from build123d import *

# Parameters (mm, degrees)
BOSS_EXTRUDE1_DEPTH = 100
SKETCH3_R           = 14.75
SKETCH3_R_2         = 2.75
BOSS_EXTRUDE2_DEPTH = 8
SKETCH4_R           = 8.075
CUT_EXTRUDE1_DEPTH  = 5.2
BOSS_EXTRUDE5_START = 11
SKETCH6_R           = 2.25
BOSS_EXTRUDE5_DEPTH = 4.5
BOSS_EXTRUDE6_DEPTH = 3


with BuildPart() as part:
    # Sketch1 → Boss-Extrude1 (new body, symmetric)
    with BuildSketch(Plane.YZ):
        with BuildLine():
            Line((-24.5, 5), (-24.5, -5))
            Line((-24.5, -5), (24.5, -5))
            Line((24.5, -5), (24.5, 5))
            Line((24.5, 5), (16.492422502, 5))
            ThreePointArc((16.492422502, 5), (0, -3), (-16.492422502, 5))
            Line((-16.492422502, 5), (-24.5, 5))
        make_face()
    extrude(amount=BOSS_EXTRUDE1_DEPTH, both=True)

    # Sketch3 → Boss-Extrude2 (add)
    with BuildSketch(Plane.XZ.offset(24.5)):
        with Locations((0, -19.75)):
            Circle(SKETCH3_R)
        with Locations((0, -19.75)):
            Circle(SKETCH3_R_2, mode=Mode.SUBTRACT)
        with BuildLine():
            Line((-14.75, -5), (-14.75, -19.75))
            ThreePointArc((-14.75, -19.75), (-10.429825021, -9.320174976), (5e-09, -5))
            Line((5e-09, -5), (-14.75, -5))
        make_face()
        with BuildLine():
            ThreePointArc((5e-09, -5), (10.429825024, -9.320174979), (14.75, -19.75))
            Line((14.75, -19.75), (14.75, -5))
            Line((14.75, -5), (5e-09, -5))
        make_face()
    boss_extrude2 = extrude(amount=-BOSS_EXTRUDE2_DEPTH)

    # Sketch4 → Cut-Extrude1 (cut)
    with BuildSketch(Plane(origin=(0, -24.5, 0), x_dir=(-1, 0, 0), z_dir=(0, -1, 0))):
        with Locations((0, 19.75)):
            Circle(SKETCH4_R)
    cut_extrude1 = extrude(amount=-CUT_EXTRUDE1_DEPTH, mode=Mode.SUBTRACT)

    # Mirror1: Boss-Extrude2, Cut-Extrude1 across plane
    add(boss_extrude2.mirror(Plane(origin=(0, 0, 0), x_dir=(0, 0, 1), z_dir=(0, -1, 0))))
    add(cut_extrude1.mirror(Plane(origin=(0, 0, 0), x_dir=(0, 0, 1), z_dir=(0, -1, 0))), mode=Mode.SUBTRACT)

    # Sketch6 → Boss-Extrude5 (add)
    with BuildSketch(Plane(origin=(0, 0, 0), x_dir=(-1, 0, 0), z_dir=(0, -1, 0)).offset(BOSS_EXTRUDE5_START)):
        with BuildLine():
            Line((87.25, 19.75), (87.25, 5))
            Line((87.25, 5), (97.75, 5))
            Line((97.75, 5), (97.75, 19.75))
            ThreePointArc((97.75, 19.75), (92.5, 25), (87.25, 19.75))
        make_face()
        with Locations((92.5, 19.75)):
            Circle(SKETCH6_R, mode=Mode.SUBTRACT)
    boss_extrude5 = extrude(amount=BOSS_EXTRUDE5_DEPTH)

    # Mirror2: Boss-Extrude5 across plane
    add(boss_extrude5.mirror(Plane(origin=(0, 0, 0), x_dir=(0, 0, 1), z_dir=(0, -1, 0))))

    # Sketch7 → Boss-Extrude6 (add)
    with BuildSketch(Plane(origin=(-100, 0, 0), x_dir=(0, -1, 0), z_dir=(-1, 0, 0))):
        with BuildLine():
            Line((24.5, 5), (16.492422502, 5))
            ThreePointArc((16.492422502, 5), (0, -3), (-16.492422502, 5))
            Line((-16.492422502, 5), (-24.5, 5))
            Line((-24.5, 5), (-24.5, -5))
            Line((-24.5, -5), (24.5, -5))
            Line((24.5, -5), (24.5, 5))
        make_face()
        with BuildLine():
            Line((-16.492422502, 5), (16.492422502, 5))
            ThreePointArc((16.492422502, 5), (0, -3), (-16.492422502, 5))
        make_face()
        with BuildLine():
            ThreePointArc((24.5, 5), (0, 13), (-24.5, 5))
            Line((-24.5, 5), (-16.492422502, 5))
            Line((-16.492422502, 5), (16.492422502, 5))
            Line((16.492422502, 5), (24.5, 5))
        make_face()
    boss_extrude6 = extrude(amount=-BOSS_EXTRUDE6_DEPTH)

    # Mirror3: Boss-Extrude6 across plane
    add(boss_extrude6.mirror(Plane(origin=(0, 0, 0), x_dir=(0, 0, 1), z_dir=(1, 0, 0))))


solid = part.part
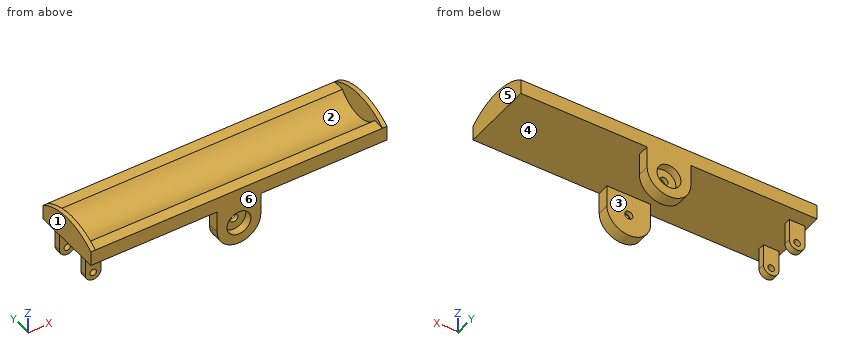
Work out the finished part from the listing and answer in its coordinate system (mm). Face numbers are marked on the shaded views. A direction names the side the tool comes from. Round coordinates to 2 decimals unless told otherwise and drop trailing zeros. Order: outer loops, then holes, each group sorted by start corner. A loop starts at its lowest first (then second) coordinate and runs counter-clockwise, first axis right, second up. Notation, with made-up numbers: M 10.25,-16.5 L 22.25,-16.5 A23 ccw 22.25,0.5 Z; hole C -5,-24 d3. An arc over 180 degrees is marked long. Put each result on its own line as item: value. Start each with the question number.
Q1. Section A-A, the plane x = -92.5 is taken. Write down the section's boundary in (y, z), and give its area (3 significant figures).
Q2. Section C-C, the plane x = -57 is taken. Write down the section's boundary in (y, z), and give its area (3 significant figures).
Q3. A tool of negligible diameter and unlimited length cuts with its end or side. For the marked faces 1, 2 and 3, from which of +Z, -Z, +X, -X, +Y, -Y can it reach the whole face along a straight path? Write none if from no direction.
Q4. Section B-B, the plane z = 7 is taken. Write down the section's boundary in (x, y), and give its area (3 significant figures).
Q5. Flat-ended cylindrical pins translate along their axes: pin 1 (6 mm diameter, centred on x = -92.5, z = -19.75, fed in from -Y); pin 2 (2.5 mm diameter, centred on y = 20, z = -13, fed in from -X); pin 3 (1.3 mm diameter, centred on y = -13.5, z = -15, fed in from -X); pin 4 (11.5 mm diameter, centred on x = -92, z = -10.5, fed in from +Y). Find the tip coordinate at first contact, or state that the pin passes through.
Q6. For a pull along Y with two mould halves and no side action, classify the marked faces 4, 5 and 6 as pulls with the +Y half, pulls with the -Y half, needs draft (parallel to the pull), parting line crosses it, or undercut.
Q7. Section D-D, the plane x = 0 is taken. Write down the section's boundary in (y, z) (3 decimals).
Q8. Straight lines are drawn through the part: L1, parallel to Z at x = 0, y = 18.65; L2, parallel to X at y = -22.8, z = -19.75 (3 decimals); L3, parallel to Y at x = 2.5, z = -13. For each, find the intervals that lie inside material, in ascending order. Write a range as [from, to].
Findings below:
1. outline: M -24.5,-5 L -15.5,-5 L -15.5,-17.5 L -11,-17.5 L -11,-5 L 11,-5 L 11,-17.5 L 15.5,-17.5 L 15.5,-5 L 24.5,-5 L 24.5,5 L 16.49,5 A21 cw -16.49,5 L -24.5,5 Z; M -15.5,-25 L -11,-25 L -11,-22 L -15.5,-22 Z; M 11,-25 L 15.5,-25 L 15.5,-22 L 11,-22 Z
1. area: 446 mm^2
2. outline: M -24.5,-5 L 24.5,-5 L 24.5,5 L 16.49,5 A21 cw -16.49,5 L -24.5,5 Z
2. area: 306 mm^2
3. face 1: +Z, -Z, -X, +Y, -Y
3. face 2: +Z
3. face 3: -Z, +X, -X
4. outline: M -100,-21.5 L -97,-21.5 L -97,21.5 L -100,21.5 Z; M 97,-21.5 L 100,-21.5 L 100,21.5 L 97,21.5 Z
4. area: 258 mm^2
5. pin 1: stops at y = -15.5
5. pin 2: stops at x = -14.75
5. pin 3: stops at x = -97.75
5. pin 4: stops at y = 24.5
6. face 4: undercut
6. face 5: needs draft
6. face 6: pulls with the -Y half
7. outline: M -24.5,-34.5 L -16.5,-34.5 L -16.5,-22.5 L -19.3,-22.5 L -19.3,-27.825 L -24.5,-27.825 Z; M -24.5,-11.675 L -19.3,-11.675 L -19.3,-17 L -16.5,-17 L -16.5,-5 L 16.5,-5 L 16.5,-17 L 19.3,-17 L 19.3,-11.675 L 24.5,-11.675 L 24.5,5 L 16.492,5 A21 cw -16.492,5 L -24.5,5 Z; M 16.5,-34.5 L 24.5,-34.5 L 24.5,-27.825 L 19.3,-27.825 L 19.3,-22.5 L 16.5,-22.5 Z
8. L1: z = [-34.5, -22.5], [-17, 5]
8. L2: x = [-14.75, -8.075], [8.075, 14.75]
8. L3: y = [-19.3, -16.5], [16.5, 19.3]
